For this review, take the finished solid that the model builds, in its own axes (mm). A direction names the side the tool comes from. Give positions to 0.01 mm unless a question says otherwise; leave off trailing zeros. Write each loop counter-clockwise with the first axis right and the second up, starting at its lowest first coordinate (ties: lowest second). Pieces come first, ordered by that corner, then holes. Notation, with made-up numbers: M 80,-2.75 L 127,-2.75 A15 ccw 127,26.25 Z; hole C 66,21.5 d2. An arc over 180 degrees is marked long. Use one line per item in the form item = value. Start each with the question number.
Q1. Consider section B-B on y = 5.5. Write out the cut boundary in (x, z).
Q2. Consider section C-C on y = -30.5. Write out the cut boundary in (x, z).
Q3. Consider section A-A on x = 22. Write out the cut boundary in (y, z), and give its area (3 significant figures).
Q4. Clearance check with flat-ended pins moving along their axes: pin 1 Ø2 at (y, z) = (-3.5, 2.5) entering from -X; pin 2 Ø6 at (x, y) = (6, -66.75) entering from +Z; pin 3 Ø1 at (x, z) = (21, 3.5) entering from +Y; pin 4 Ø2 at (y, z) = (-40.5, 2.5) entering from -X. State where each tip first meets the part, or that it passes through.
Q5. Mouldability with a two-part tool opening along Y and no side actions: class faces 4 (the flat face through (26, -68.255, 2)), 5 (the flat face through (30.336, -55.579, 1.972)), 6 (the flat face through (18, -0.5, 2)), 7 (the flat face through (34, 7.005, 2)) as released by +Y, released by -Y, zero draft, split by the parting line, or undercut.
Q6. Tool access review of faces 1 (the flat face through (10, -68.255, 2)), 2 (the flat face through (3, 0, 2)), 3 (the flat face through (10.378, -4, 2)): name each direction out of +Z, -Z, +X, -X, +Y, -Y from which nothing blocks a thin tool from reaching the whole face with its end or side.
Q7. For probe 1 along X at (y, z) = (5.5, 2.2); probe 2 along X at (y, z) = (-2, 1.15); probe 3 along X at (y, z) = (3.5, 2.2), list the stretches that pass through material, from the lowest coordinate up. Write a range as [from, to].
```python
from build123d import *

# Parameters (mm, degrees)
F0_W     = 15.25
F0_H     = 6.25
F1_DEPTH = 4


with BuildPart() as f1:
    # F0 (on Top) → F1 (new body)
    with BuildSketch(Plane.XY):
        with BuildLine():
            ThreePointArc((8, 7.004538), (6.003411, 3), (4.006822, 7.004538))
            Line((4.006822, 7.004538), (0, 7.004538))
            Line((0, 7.004538), (0, 0))
            Line((0, 0), (5.603411, 0))
            Line((5.603411, 0), (5.603411, -7.25))
            Line((5.603411, -7.25), (11.503411, -13.15))
            Line((11.503411, -13.15), (11.503411, -49.746589))
            Line((11.503411, -49.746589), (0, -61.25))
            Line((0, -61.25), (0, -68.254538))
            Line((0, -68.254538), (4.006822, -68.254538))
            ThreePointArc((4.006822, -68.254538), (6.003411, -64.25), (8, -68.254538))
            Line((8, -68.254538), (12.006822, -68.254538))
            ThreePointArc((12.006822, -68.254538), (14.003411, -64.25), (16, -68.254538))
            Line((16, -68.254538), (20.006822, -68.254538))
            ThreePointArc((20.006822, -68.254538), (22.003411, -64.25), (24, -68.254538))
            Line((24, -68.254538), (28.006822, -68.254538))
            ThreePointArc((28.006822, -68.254538), (30.003411, -64.25), (32, -68.254538))
            Line((32, -68.254538), (36.006822, -68.254538))
            Line((36.006822, -68.254538), (36.006822, -61.25))
            Line((36.006822, -61.25), (24.503411, -49.746589))
            Line((24.503411, -49.746589), (24.503411, -13.15))
            Line((24.503411, -13.15), (30.403411, -7.25))
            Line((30.403411, -7.25), (30.403411, 0))
            Line((30.403411, 0), (36.006822, 0))
            Line((36.006822, 0), (36.006822, 7.004538))
            Line((36.006822, 7.004538), (32, 7.004538))
            ThreePointArc((32, 7.004538), (30.003411, 3), (28.006822, 7.004538))
            Line((28.006822, 7.004538), (24, 7.004538))
            ThreePointArc((24, 7.004538), (22.003411, 3), (20.006822, 7.004538))
            Line((20.006822, 7.004538), (16, 7.004538))
            ThreePointArc((16, 7.004538), (14.003411, 3), (12.006822, 7.004538))
            Line((12.006822, 7.004538), (8, 7.004538))
        make_face()
        with Locations((18.003411, -3.625)):
            Rectangle(F0_W, F0_H, mode=Mode.SUBTRACT)
    extrude(amount=F1_DEPTH)


solid = f1.part
```
Working result:
q1.outline = M 0,0 L 3.5,0 L 3.5,4 L 0,4 Z; M 8.5,0 L 11.5,0 L 11.5,4 L 8.5,4 Z; M 16.5,0 L 19.5,0 L 19.5,4 L 16.5,4 Z; M 24.5,0 L 27.5,0 L 27.5,4 L 24.5,4 Z; M 32.5,0 L 36.01,0 L 36.01,4 L 32.5,4 Z
q2.outline = M 11.5,0 L 24.5,0 L 24.5,4 L 11.5,4 Z
q3.outline = M -64.25,0 L -6.75,0 L -6.75,4 L -64.25,4 Z; M -0.5,0 L 3,0 L 3,4 L -0.5,4 Z
q3.area = 244 mm²
q4.pin_1 = 5.6
q4.pin_2 = 4
q4.pin_3 = 3.5
q4.pin_4 = 11.5
q5.face_4 = released by -Y
q5.face_5 = undercut
q5.face_6 = undercut
q5.face_7 = released by +Y
q6.face_1 = +Z, -Z, +X, -X, -Y
q6.face_2 = +Z, -Z, -X
q6.face_3 = +Z, -Z
q7.probe_1 = [0, 3.5], [8.5, 11.5], [16.5, 19.5], [24.5, 27.5], [32.5, 36.01]
q7.probe_2 = [5.6, 10.38], [25.63, 30.4]
q7.probe_3 = [0, 4.5], [7.5, 12.5], [15.5, 20.5], [23.5, 28.5], [31.5, 36.01]
